```python
from build123d import *

# Parameters (mm, degrees)
CROQUIS3_R              = 6.36
SALIENTE_EXTRUIR2_DEPTH = 39.6
CROQUIS4_R              = 3.175
CORTAR_EXTRUIR1_DEPTH   = 19.3
CROQUIS6_W              = 3.95
CROQUIS6_H              = 2.393963958
CORTAR_EXTRUIR3_DEPTH   = 20
CHAFL_N1_SIZE           = 0.95
CHAFL_N1_SIZE2          = 1
CHAFL_N2_SIZE           = 0.5


with BuildPart() as part:
    # Croquis3 → Saliente-Extruir2 (new body)
    with BuildSketch(Plane.XY):
        Circle(CROQUIS3_R)
    extrude(amount=-SALIENTE_EXTRUIR2_DEPTH)

    # Croquis4 → Cortar-Extruir1 (cut)
    with BuildSketch(Plane.XY):
        Circle(CROQUIS4_R)
    extrude(amount=-CORTAR_EXTRUIR1_DEPTH, mode=Mode.SUBTRACT)

    # Croquis6 → Cortar-Extruir3 (cut)
    with BuildSketch(Plane(origin=(0, 0, -39.6), x_dir=(-1, 0, 0), z_dir=(0, 0, -1))):
        with Locations((-0.01, 5.546981979)):
            Rectangle(CROQUIS6_W, CROQUIS6_H)
    extrude(amount=-CORTAR_EXTRUIR3_DEPTH, mode=Mode.SUBTRACT)

    # Chaflán1
    chafl_n1_edges = [part.edges().sort_by_distance(p)[0] for p in [
        (-3.738462251, -5.145240519, -39.6),
    ]]
    chafl_n1_side = [part.faces().sort_by_distance(p)[0] for p in [
        (-0.000560241, -0.334162106, -39.6),
    ]]
    chamfer(chafl_n1_edges, length=CHAFL_N1_SIZE, length2=CHAFL_N1_SIZE2, reference=chafl_n1_side[0])

    # Chaflán2
    chafl_n2_edges = [part.edges().sort_by_distance(p)[0] for p in [
        (-3.175, 0, 0),
    ]]
    chamfer(chafl_n2_edges, length=CHAFL_N2_SIZE)


solid = part.part
```
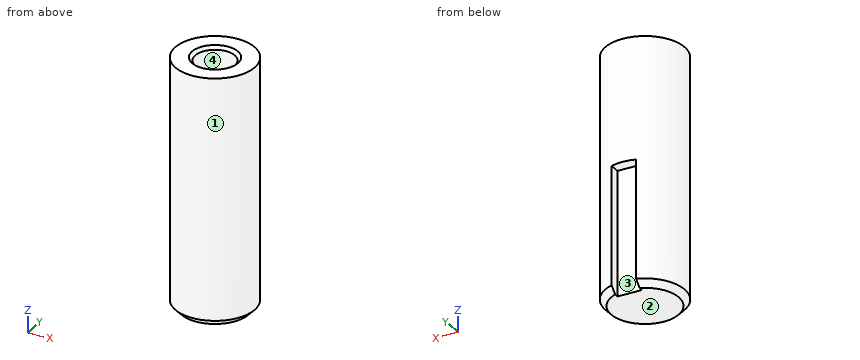
Input: part model. Units: mm. Frame: model coordinates. Face numbers are marked on the shaded views. Give positions to 0.01 mm unless a question says otherwise; leave off trailing zeros. Order: outer loops, then holes, each group sorted by start corner. A loop starts at its lowest first (then second) coordinate and runs counter-clockwise, first axis right, second up. Notation, with made-up numbers: (-2.75, 59.5) -> (44.25, 59.5) arc R17 cw to (44.25, 66.5) -> close; hole circle Ø3 at (-13, 81.25). An arc over 180 degrees is marked (long way). Write each question's results on one line, items separated by ' | '. Start each with the question number.
Item 1: Mould query, pull axis Y, two halves, no side actions, for the marked faces 1, 2, 3 and 4. Classes: pulls with the +Y half, pulls with the -Y half, needs draft (parallel to the pull), parting line crosses it, or undercut.
Item 2: Cut plane A-A on x = 0. Return the cut outline in (y, z) (3 decimals).
Item 3: Line query: line 1 (Y direction, x = 0, z = -5) (3 decimals); line 2 (X direction, y = -0.5, z = -1.5); line 3 (X direction, y = 2.75, z = -15). Output: solid intervals per line, ascending.
Item 4: Cut plane B-B on z = -32.5. Return the cut outline in (x, y) (3 decimals).
Item 5: Contact query for flat-ended pins moving along their axis: P1, Ø3, axis at x = -4, z = -17.5, coming from the +Y side; P2, Ø1.9, axis at x = 0.5, y = 0, coming from the +Z side; P3, Ø1.4, axis at y = 5, z = -30.5, coming from the -X side. Output: stop coordinate, or through.
Established:
1) face 1: parting line crosses it | face 2: needs draft | face 3: pulls with the +Y half | face 4: undercut
2) outline: (-6.36, -38.6) -> (-5.41, -39.6) -> (4.35, -39.6) -> (4.35, -19.6) -> (6.36, -19.6) -> (6.36, 0) -> (3.675, 0) -> (3.175, -0.5) -> (3.175, -19.3) -> (-3.175, -19.3) -> (-3.175, -0.5) -> (-3.675, 0) -> (-6.36, 0) -> close
3) line 1: -6.36 to -3.175, 3.175 to 6.36 | line 2: -6.34 to -3.14, 3.14 to 6.34 | line 3: -5.73 to -1.59, 1.59 to 5.73
4) outline: (-1.965, 4.35) -> (-1.965, 6.049) arc R6.36 ccw (long way) to (1.985, 6.042) -> (1.985, 4.35) -> close
5) P1: y = 5.85 | P2: z = -19.3 | P3: x = -4.69
